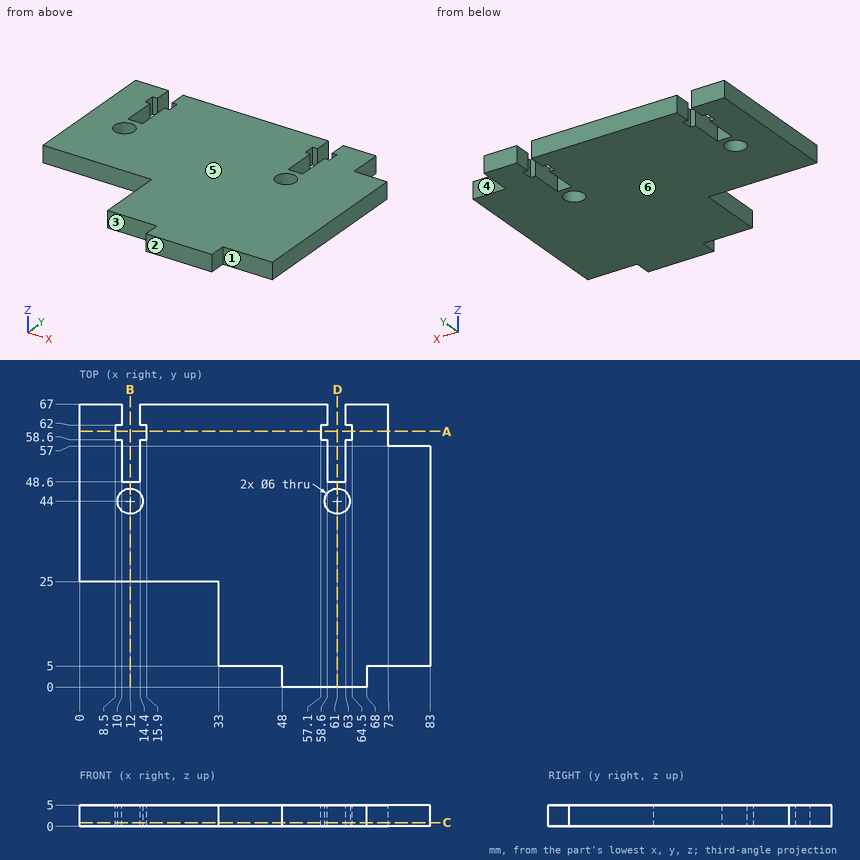
Can you work these out from the drawing? Everything is in mm from the part's minimum corner. A direction names the side the tool comes from. Coordinates: 2 decimals unless noted, no trailing zeros. Order: outer loops, then holes, each group sorted by start corner. A loop starts at its lowest first (then second) coordinate and runs counter-clockwise, first axis right, second up. Notation, with made-up numbers: (24.5, 47) -> (66.5, 47) arc R16 cw to (66.5, 60) -> close; hole circle Ø11 at (20.25, 11). An arc over 180 degrees is marked (long way). Return JSON: item names as keys, results as strings.
1) If we section it at D-D on x = 61: List the corners of the cut face in (y, z) for me, plus the area to 3 significant figures.
Conclusion:
{"outline": "(0, 0) -> (41, 0) -> (41, 5) -> (0, 5) -> close; (47, 0) -> (48.6, 0) -> (48.6, 5) -> (47, 5) -> close", "area": "213 mm²"}
2) If we section it at B-B on x = 12: List the corners of the cut face in (y, z) for me, plus the area to 3 significant figures.
Conclusion:
{"outline": "(25, 0) -> (41, 0) -> (41, 5) -> (25, 5) -> close; (47, 0) -> (48.6, 0) -> (48.6, 5) -> (47, 5) -> close", "area": "88.0 mm²"}
3) If we section it at A-A on y = 60.5: List the corners of the cut face in (x, z) for me.
Conclusion:
{"outline": "(0, 0) -> (8.5, 0) -> (8.5, 5) -> (0, 5) -> close; (15.9, 0) -> (57.1, 0) -> (57.1, 5) -> (15.9, 5) -> close; (64.5, 0) -> (73, 0) -> (73, 5) -> (64.5, 5) -> close"}
4) Thinking about a two-plate mould opening in Z: for the marked faces 4, 5 and 6, which applies, +Z half, -Z half, draft (parallel to the pull), parting line (faces both ways), or undercut?
Conclusion:
{"face 4": "draft", "face 5": "+Z half", "face 6": "-Z half"}
5) I'm going to push flat-ended pins straight in: P1, Ø2, axis at x = 11.5, z = 3, coming from the +Y side; P2, Ø1.5, axis at y = 2, z = 2, coming from the -X side; P3, Ø2.5, axis at x = 12.5, z = 3.5, coming from the -Y side. Where does each tip first touch, or does it pass through?
Conclusion:
{"P1": "stops at y = 48.6", "P2": "stops at x = 48", "P3": "stops at y = 25"}
6) On a 3-axis mill with a long thin cutter (end or side, diameter ignored), from which of +Z, -Z, +X, -X, +Y, -Y can I reach the whole of each face in a straight line? I mean the marked faces 1, 2 and 3. Say none if no direction works.
Conclusion:
{"face 1": "+Z, -Z, +X, -Y", "face 2": "+Z, -Z, +X, -X, -Y", "face 3": "+Z, -Z, -X, -Y"}
7) If I drill on probe 1 along X at (y, z) = (62.5, 2.05); probe 2 along Y at (x, z) = (12, 1.45); probe 3 along Y at (x, z) = (61, 3.65), over which ranges is the centre line in solid material (lowest first)?
Conclusion:
{"probe 1": "x = 0 to 10, 14.4 to 58.6, 63 to 73", "probe 2": "y = 25 to 41, 47 to 48.6", "probe 3": "y = 0 to 41, 47 to 48.6"}
8) If we section it at C-C on z = 0.9: State how many separate pieces and enclosed holes the cut face has, plus the area to 3 significant figures.
Conclusion:
{"separate pieces": "1", "enclosed holes": "2", "area": "4,250 mm²"}
